Here's how the part is built. I have some questions about the finished solid (model axes, mm). A direction names the side the tool comes from. Give positions to 0.01 mm unless a question says otherwise; leave off trailing zeros. Write each loop counter-clockwise with the first axis right and the second up, starting at its lowest first coordinate (ties: lowest second). Pieces come first, ordered by that corner, then holes. Notation, with made-up numbers: (7, 40.5) -> (64, 40.5) arc R14 ccw to (64, 59.5) -> close; hole circle Ø5 at (-9, -36). An arc over 180 degrees is marked (long way). Put each result on its own line as item: value. Start each with the question number.
from build123d import *

# Parameters (mm, degrees)
SKETCH5_R               = 22.843403387
SKETCH5_R_2             = 13.335
BOSS_EXTRUDE2_DEPTH     = 3.175
SKETCH8_R               = 22.843403387
SKETCH8_R_2             = 19.668403387
BOSS_EXTRUDE3_DEPTH     = 10.16
CUT_EXTRUDE2_DEPTH      = 35.949454799
CUT_EXTRUDE2_DEPTH_BACK = 35.949454799
SKETCH9_R               = 1.905
SKETCH11_R              = 22.843403387
SKETCH11_R_2            = 21.59
CUT_EXTRUDE3_DEPTH      = 3.175
SKETCH12_R              = 30.48
SKETCH12_R_2            = 21.59
BOSS_EXTRUDE4_DEPTH     = 3.175
CUT_EXTRUDE4_DEPTH      = 45.286413266
CUT_EXTRUDE4_DEPTH_BACK = 45.286413266
SKETCH13_W              = 6.35
SKETCH13_H              = 8.89
SKETCH14_R              = 4.445
CUT_EXTRUDE5_DEPTH      = 1.4478
SKETCH15_R              = 1.5875
BOSS_EXTRUDE5_DEPTH     = 13.21
SKETCH16_R              = 1.27
CUT_EXTRUDE6_DEPTH      = 3.175


with BuildPart() as part:
    # Loft1: read off the stored shape, not the designer's step
    # Loft1: loft between two sections, ruled curve by curve
    loft1_from = [
        Edge.make_bspline([(10.081206282, 0, 5.386481216), (20.854168715, 0, -14.775931349), (0.69175615, 0, -25.548893781), (-10.081206282, 0, -5.386481216), (-20.854168715, 0, 14.775931349), (-0.69175615, 0, 25.548893781), (10.081206282, 0, 5.386481216)], [0, 0, 0, 0, 0.5, 0.5, 0.5, 1, 1, 1, 1], 3, [1, 0.333333333, 0.333333333, 1, 0.333333333, 0.333333333, 1]),
    ]
    loft1_to = [
        Edge.make_bspline([(16.298540151, 3.175, 2.633949306), (21.566438762, 3.175, -29.963130997), (-11.03064154, 3.175, -35.231029608), (-16.298540151, 3.175, -2.633949306), (-21.566438762, 3.175, 29.963130997), (11.03064154, 3.175, 35.231029608), (16.298540151, 3.175, 2.633949306)], [0, 0, 0, 0, 0.5, 0.5, 0.5, 1, 1, 1, 1], 3, [1, 0.333333333, 0.333333333, 1, 0.333333333, 0.333333333, 1]),
    ]
    loft1 = Solid(Shell([*[Face.make_surface_from_curves(loft1_from[k], loft1_to[k]) for k in range(1)], Face(Wire(loft1_from)), Face(Wire(loft1_to))]))
    add(loft1)

    # Cut-Loft1: read off the stored shape, not the designer's step
    # Cut-Loft1: loft between two sections, ruled curve by curve
    cut_loft1_from = [
        Edge.make_bspline([(11.717693295, 3.175, 6.365366356), (-1.013039416, 3.175, 29.800752946), (-24.448426006, 3.175, 17.070020235), (-11.717693295, 3.175, -6.365366356), (1.013039416, 3.175, -29.800752946), (24.448426006, 3.175, -17.070020235), (11.717693295, 3.175, 6.365366356)], [0, 0, 0, 0, 0.5, 0.5, 0.5, 1, 1, 1, 1], 3, [1, 0.333333333, 0.333333333, 1, 0.333333333, 0.333333333, 1]),
    ]
    cut_loft1_to = [
        Edge.make_bspline([(5.259513685, 0, 8.692704746), (-12.125895806, 0, 19.211732116), (-22.644923177, 0, 1.826322624), (-5.259513685, 0, -8.692704746), (12.125895806, 0, -19.211732116), (22.644923177, 0, -1.826322624), (5.259513685, 0, 8.692704746)], [0, 0, 0, 0, 0.5, 0.5, 0.5, 1, 1, 1, 1], 3, [1, 0.333333333, 0.333333333, 1, 0.333333333, 0.333333333, 1]),
    ]
    cut_loft1 = Solid(Shell([*[Face.make_surface_from_curves(cut_loft1_from[k], cut_loft1_to[k]) for k in range(1)], Face(Wire(cut_loft1_from)), Face(Wire(cut_loft1_to))]))
    add(cut_loft1, mode=Mode.SUBTRACT)

    # Sketch5 → Boss-Extrude2 (add)
    with BuildSketch(Plane(origin=(0, 3.175, 0), x_dir=(1, 0, 0), z_dir=(0, 1, 0))):
        with Locations(Location((0, 0, 0), (0, 0, 270))):
            Circle(SKETCH5_R)
        with Locations(Location((0, 0, 0), (0, 0, 270))):
            Circle(SKETCH5_R_2, mode=Mode.SUBTRACT)
    extrude(amount=-BOSS_EXTRUDE2_DEPTH)

    # Sketch10 → Revolve4 (revolve)
    with BuildSketch(Plane.XY):
        Polygon((-13.335, 1.305724577), (-10.16, 0), (-13.335, 0), align=None)
    revolve(axis=Axis((0, -10.16, 0), (0, 1, 0)))

    # Sketch8 → Boss-Extrude3 (add)
    with BuildSketch(Plane(origin=(0, 0, 0), x_dir=(-1, 0, 0), z_dir=(0, -1, 0))):
        with Locations(Location((0, 0, 0), (0, 0, 270))):
            Circle(SKETCH8_R)
        with Locations(Location((0, 0, 0), (0, 0, 90))):
            Circle(SKETCH8_R_2, mode=Mode.SUBTRACT)
    extrude(amount=BOSS_EXTRUDE3_DEPTH)

    # Sketch9 → Cut-Extrude2 (cut, two sides: drawn at the far end of the back side and taken through both)
    with BuildSketch(Plane(origin=(0, 3.175, 0), x_dir=(1, 0, 0), z_dir=(0, 1, 0)).offset(-CUT_EXTRUDE2_DEPTH_BACK)):
        with Locations(Location((19.033403387, 0, 0), (0, 0, 270))):
            Circle(SKETCH9_R)
        with Locations(Location((-19.033403387, 0, 0), (0, 0, 270))):
            Circle(SKETCH9_R)
    extrude(amount=CUT_EXTRUDE2_DEPTH + CUT_EXTRUDE2_DEPTH_BACK, mode=Mode.SUBTRACT)

    # Sketch11 → Cut-Extrude3 (cut)
    with BuildSketch(Plane(origin=(0, 3.175, 0), x_dir=(1, 0, 0), z_dir=(0, 1, 0))):
        with Locations(Location((0, 0, 0), (0, 0, 270))):
            Circle(SKETCH11_R)
        with Locations(Location((0, 0, 0), (0, 0, 270))):
            Circle(SKETCH11_R_2, mode=Mode.SUBTRACT)
    extrude(amount=-CUT_EXTRUDE3_DEPTH, mode=Mode.SUBTRACT)

    # Sketch12 → Boss-Extrude4 (add)
    with BuildSketch(Plane(origin=(0, 0, 0), x_dir=(1, 0, 0), z_dir=(0, 1, 0))):
        with Locations(Location((0, 0, 0), (0, 0, 270))):
            Circle(SKETCH12_R)
        with Locations(Location((0, 0, 0), (0, 0, 270))):
            Circle(SKETCH12_R_2, mode=Mode.SUBTRACT)
    extrude(amount=-BOSS_EXTRUDE4_DEPTH)

    # Sketch13 → Cut-Extrude4 (cut, two sides: drawn at the far end of the back side and taken through both)
    with BuildSketch(Plane(origin=(0, 0, 0), x_dir=(1, 0, 0), z_dir=(0, 1, 0)).offset(-CUT_EXTRUDE4_DEPTH_BACK)):
        with Locations((0, -26.035)):
            Rectangle(SKETCH13_W, SKETCH13_H)
    extrude(amount=CUT_EXTRUDE4_DEPTH + CUT_EXTRUDE4_DEPTH_BACK, mode=Mode.SUBTRACT)

    # Sketch14 → Cut-Extrude5 (cut)
    with BuildSketch(Plane(origin=(0, 3.175, 0), x_dir=(1, 0, 0), z_dir=(0, 1, 0))):
        with Locations((-19.033403387, 0)):
            Circle(SKETCH14_R)
        with Locations((19.033403387, 0)):
            Circle(SKETCH14_R)
    extrude(amount=-CUT_EXTRUDE5_DEPTH, mode=Mode.SUBTRACT)

    # Sketch15 → Boss-Extrude5 (add)
    with BuildSketch(Plane.XZ):
        with Locations(Location((10.276942125, -12.684023832, 0), (0, 0, 90))):
            Circle(SKETCH15_R)
        with Locations(Location((-10.719763295, -12.312054049, 0), (0, 0, 90))):
            Circle(SKETCH15_R)
    extrude(amount=BOSS_EXTRUDE5_DEPTH)

    # Sketch16 → Cut-Extrude6 (cut)
    with BuildSketch(Plane(origin=(0, -13.21, 0), x_dir=(-1, 0, 0), z_dir=(0, -1, 0))):
        with Locations(Location((10.719763295, 12.312054049, 0), (0, 0, 90))):
            Circle(SKETCH16_R)
        with Locations(Location((-10.276942125, 12.684023832, 0), (0, 0, 90))):
            Circle(SKETCH16_R)
    extrude(amount=-CUT_EXTRUDE6_DEPTH, mode=Mode.SUBTRACT)


solid = part.part
1) I'm going to push flat-ended pins straight in: pin 1 Ø2 at (x, y) = (-14, -4) entering from -Z; pin 2 Ø1.5 at (y, z) = (-6.5, -13) entering from -X; pin 3 Ø4 at (x, y) = (14, -2) entering from -Z. Where does each tip first touch, or does it pass through?
2) Thinking about a two-plate mould opening in Z: for faces 1 (the flat face through (-3.175, -3, 25)), 2 (the cylindrical face through (1.296, -1.565, -30.452)), 3 (the cylindrical face through (14.59, 2.46, -0.13)), which applies, released by +Z, released by -Z, zero draft, split by the parting line, or undercut?
3) I want a section at D-D, the plane z = -15.5. Write out the boundary of the cut face in (x, y) (3 decimals), and give its area (3 significant figures).
4) I want a section at A-A, the plane y = -6.5. Write out the boundary of the cut face in (x, z) (1 decimal), and give its area (3 significant figures).
5) I want a section at C-C, the plane y = -11. Write out the boundary of the cut face in (x, z) (1 decimal).
6) Which directions (+Z, -Z, +X, -X, +Y, -Y) give clear straight access to the entire face, cutting with the end or side of a thin tool? Please do faces 4 (the cylindrical face through (-20.893, -4.3, -0.413)), 5 (the flat face through (17, 1.727, 1)), 6 (the flat face through (10, 3.175, -10)), 7 (the flat face through (3.175, -3, 25)), 8 (the cylindrical face through (10.658, -11.645, -13.895)).
7) I need wall thicknesses on probe 1 along X at (y, z) = (-0.5, 0); probe 2 along X at (y, z) = (-7, 0); probe 3 along Y at (x, z) = (-26, 5.5) (3 decimals). Which ranges of each line are inside material? Lowest first, please.
8) I want a section at B-B, the plane z = 0. State how many separate pieces and enclosed holes the cut face has, and give its area (3 significant figures).
Established:
1. pin 1: stops at z = -27.36
1. pin 2: stops at x = -19.28
1. pin 3: stops at z = -28.02
2. face 1: zero draft
2. face 2: split by the parting line
2. face 3: undercut
3. outline: (-26.245, -3.175) -> (-16.78, -3.175) -> (-16.78, -10.16) -> (-12.108, -10.16) -> (-12.108, 0) -> (12.108, 0) -> (12.108, -10.16) -> (16.78, -10.16) -> (16.78, -3.175) -> (26.245, -3.175) -> (26.245, 0) -> (15.029, 0) -> (15.029, 3.175) -> (-15.029, 3.175) -> (-15.029, 0) -> (-26.245, 0) -> close
3. area: 250 mm2
4. outline: circle Ø3.2 at (-10.7, -12.3); (-3.2, 21.6) -> (-3.2, 22.6) arc R22.8 ccw (long way) to (3.2, 22.6) -> (3.2, 21.6) -> close; circle Ø3.2 at (10.3, -12.7); hole (-19.6, -1.8) arc R19.7 ccw to (19.6, -1.8) arc R1.9 ccw to (19.6, 1.8) arc R19.7 ccw to (-19.6, 1.8) arc R1.9 ccw to start
4. area: 426 mm2
5. outline: circle Ø3.2 at (-10.7, -12.3); circle Ø3.2 at (10.3, -12.7); hole circle Ø2.5 at (-10.7, -12.3); hole circle Ø2.5 at (10.3, -12.7)
6. face 4: +Y, -Y
6. face 5: +Y
6. face 6: +Z, -Z, +X, -X, +Y
6. face 7: +Z, +Y, -Y
6. face 8: -Y
7. probe 1: x = -30.48 to -20.94, 20.94 to 30.48
7. probe 2: x = -22.84 to -20.94, 20.94 to 22.84
7. probe 3: y = -3.175 to 0
8. separate pieces: 4
8. enclosed holes: 0
8. area: 118 mm2
